Verification items for the finished model (mm, model axes). Face numbers are marked on the shaded views. Coordinates: 2 decimals unless noted, no trailing zeros. Loops run counter-clockwise (first coordinate to the right, second up) from the corner with the lowest first, then second, coordinate; pieces in that order, holes last. Notation, with made-up numbers: (-11, 33.25) - (22, 33.25) arc R23 cw to (22, 45.25) - close; hole circle Ø9 at (15, 38.5). An arc over 180 degrees is marked (long way). One line per item, written item: value. Start each with the question number.
(1) Thickness scan on probe 1 along Y at (x, z) = (8.5, 0) (1 decimal); probe 2 along Y at (x, z) = (12.5, 0) (1 decimal); probe 3 along Z at (x, y) = (7.5, 17.5). Record the ranges inside material, lowest first. Write a range as [from, to].
(2) Draft check along Y on the marked faces 1 and 2. Enter one of: +Y half, -Y half, draft (parallel to the pull), parting line (faces both ways), or undercut.
(3) Section check A-A (z = 0). Record the boundary of the cut face in (x, y) (1 decimal), plus the area to 3 significant figures.
(4) Section check B-B (x = 12.5). Count the separate pieces of the cut face and the enclosed holes in it, plus the area to 3 significant figures.
(5) Gauge pin test, flat ends, axial feed: P1, Ø5, axis at x = 10, z = 17.5, coming from the -Y side; P2, Ø12, axis at x = 7.5, z = 9, coming from the -Y side; P3, Ø12, axis at x = 2.5, y = 12, coming from the +Z side; P4, Ø8.5, axis at y = 0, z = 0, coming from the -X side. Record the tip position at first contact, or that the pin passes through.
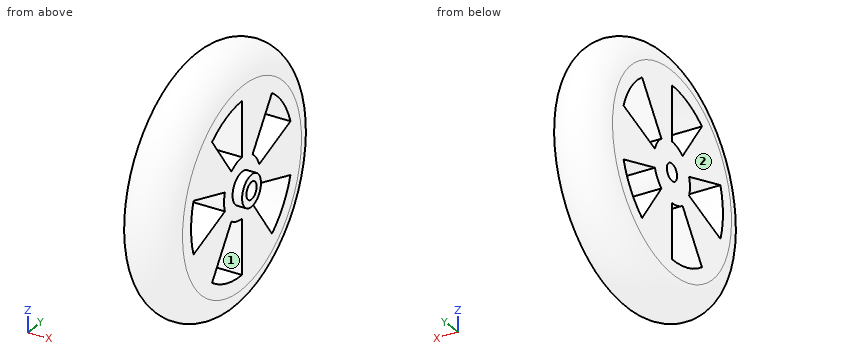
```python
from build123d import *

# Parameters (mm, degrees)
SKETCH2_R          = 2.7
CUT_EXTRUDE1_DEPTH = 61.000000133
CUT_EXTRUDE2_DEPTH = 61.000000133


with BuildPart() as part:
    # Sketch1 → Revolve1 (revolve)
    with BuildSketch(Plane.XY, mode=Mode.PRIVATE) as revolve1_sk:
        with BuildLine():
            Line((0, 31.5), (0, 0))
            Line((0, 0), (20, 0))
            Line((20, 0), (20, 5))
            Line((20, 5), (17, 5))
            Line((17, 5), (17, 31.5))
            ThreePointArc((17, 31.5), (8.5, 40), (0, 31.5))
        make_face()
    revolve(revolve1_sk.sketch.rotate(Axis((0, 0, 0), (1, 0, 0)), 90), axis=Axis((0, 0, 0), (1, 0, 0)))

    # Sketch2 → Cut-Extrude1 (cut, through all)
    with BuildSketch(Plane(origin=(0, 0, 0), x_dir=(0, 0, -1), z_dir=(1, 0, 0))):
        Circle(SKETCH2_R)
    extrude(amount=CUT_EXTRUDE1_DEPTH, mode=Mode.SUBTRACT)

    # Sketch3 → Cut-Extrude2 (cut, through all)
    with BuildSketch(Plane(origin=(0, 0, 0), x_dir=(0, 0, -1), z_dir=(1, 0, 0))):
        with BuildLine():
            Line((-21.833346136, 15.862854496), (-7.705886871, 5.598654528))
            ThreePointArc((-7.705886871, 5.598654528), (-5.598654528, 7.705886871), (-2.943386871, 9.058813318))
            Line((-2.943386871, 9.058813318), (-8.339596136, 25.666637734))
            ThreePointArc((-8.339596136, 25.666637734), (-15.862854496, 21.833346136), (-21.833346136, 15.862854496))
        make_face()
        with BuildLine():
            Line((8.339596136, 25.666637734), (2.943386871, 9.058813318))
            ThreePointArc((2.943386871, 9.058813318), (5.598654528, 7.705886871), (7.705886871, 5.598654528))
            Line((7.705886871, 5.598654528), (21.833346136, 15.862854496))
            ThreePointArc((21.833346136, 15.862854496), (15.862854496, 21.833346136), (8.339596136, 25.666637734))
        make_face()
        with BuildLine():
            Line((26.9875, 0), (9.525, 0))
            ThreePointArc((9.525, 0), (9.058813318, -2.943386871), (7.705886871, -5.598654528))
            Line((7.705886871, -5.598654528), (21.833346136, -15.862854496))
            ThreePointArc((21.833346136, -15.862854496), (25.666637734, -8.339596136), (26.9875, 0))
        make_face()
        with BuildLine():
            Line((8.339596136, -25.666637734), (2.943386871, -9.058813318))
            ThreePointArc((2.943386871, -9.058813318), (0, -9.525), (-2.943386871, -9.058813318))
            Line((-2.943386871, -9.058813318), (-8.339596136, -25.666637734))
            ThreePointArc((-8.339596136, -25.666637734), (0, -26.9875), (8.339596136, -25.666637734))
        make_face()
        with BuildLine():
            Line((-21.833346136, -15.862854496), (-7.705886871, -5.598654528))
            ThreePointArc((-7.705886871, -5.598654528), (-9.058813318, -2.943386871), (-9.525, 0))
            Line((-9.525, 0), (-26.9875, 0))
            ThreePointArc((-26.9875, 0), (-25.666637734, -8.339596136), (-21.833346136, -15.862854496))
        make_face()
    extrude(amount=CUT_EXTRUDE2_DEPTH, mode=Mode.SUBTRACT)


solid = part.part
```
Responses:
1. probe 1: y = [-40, -27], [-9.5, -2.7], [2.7, 40]
1. probe 2: y = [-39, -27], [-9.5, -2.7], [2.7, 39]
1. probe 3: z = [-35.9, -20.54], [-5.69, 5.69], [20.54, 35.9]
2. face 1: undercut
2. face 2: draft
3. outline: (0, -31.5) arc R8.5 ccw to (17, -31.5) - (17, -27) - (0, -27) - close; (0, -9.5) - (17, -9.5) - (17, -5) - (20, -5) - (20, -2.7) - (0, -2.7) - close; (0, 2.7) - (20, 2.7) - (20, 5) - (17, 5) - (17, 31.5) arc R8.5 ccw to (0, 31.5) - close
3. area: 923 mm²
4. separate pieces: 1
4. enclosed holes: 6
4. area: 3,750 mm²
5. P1: stops at y = -37
5. P2: stops at y = -39.88
5. P3: stops at z = 39.05
5. P4: stops at x = 0
